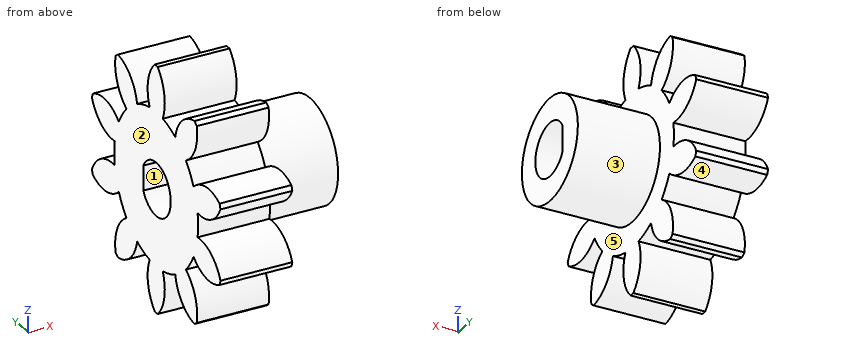
```python
from build123d import *

# Parameters (mm, degrees)
BASPROSKE_W         = 15
BASPROSKE_H         = 12
TOOTHCUT_DEPTH      = 23.649503306
TEETHCUTS_COUNT     = 10
TEETHCUTS_ANGLE     = 324
BORSKE_R            = 0.45
BORE_DEPTH          = 50.0000508
SKETCH1_R           = 0.45
CUT_EXTRUDE1_DEPTH  = 15
CUT_EXTRUDE2_DEPTH  = 8
SKETCH6_R           = 5
BOSS_EXTRUDE1_DEPTH = 8


with BuildPart() as part:
    # BasProSke → Base-Revolve (revolve)
    with BuildSketch(Plane(origin=(0, 0, 0), x_dir=(1, 0, 0), z_dir=(0, 1, 0)), mode=Mode.PRIVATE) as base_revolve_sk:
        with Locations((7.5, 6)):
            Rectangle(BASPROSKE_W, BASPROSKE_H)
    revolve(base_revolve_sk.sketch.rotate(Axis((-10, 0, 0), (1, 0, 0)), 180), axis=Axis((-10, 0, 0), (1, 0, 0)))

    # TooCutSke → ToothCut (cut, through all)
    with BuildSketch(Plane(origin=(0, 0, 0), x_dir=(0, 0, -1), z_dir=(1, 0, 0))):
        with BuildLine():
            ThreePointArc((1.173662691, 7.406586048), (0, 7.499), (-1.173662691, 7.406586048))
            ThreePointArc((-1.173662691, 7.406586048), (-1.668191438, 9.834565786), (-3.497907776, 11.50542856))
            ThreePointArc((-3.497907776, 11.50542856), (0, 12.0254), (3.497907776, 11.50542856))
            ThreePointArc((3.497907776, 11.50542856), (1.668191438, 9.834565786), (1.173662691, 7.406586048))
        make_face()
    toothcut = extrude(amount=TOOTHCUT_DEPTH, mode=Mode.SUBTRACT)

    # TeethCuts: ToothCut ×10 about axis
    teethcuts_axis = Axis((-10, 0, 0), (1, 0, 0))
    for i in range(1, TEETHCUTS_COUNT):
        add(toothcut.rotate(teethcuts_axis, i * TEETHCUTS_ANGLE / (TEETHCUTS_COUNT - 1)), mode=Mode.SUBTRACT)

    # BorSke → Bore (cut, symmetric)
    with BuildSketch(Plane(origin=(0, 0, 0), x_dir=(0, 0, -1), z_dir=(1, 0, 0))):
        with Locations(Location((0, 0, 0), (0, 0, 180))):
            Circle(BORSKE_R)
    extrude(amount=BORE_DEPTH, both=True, mode=Mode.SUBTRACT)

    # Sketch1 → Cut-Extrude1 (cut)
    with BuildSketch(Plane.ZY):
        with BuildLine():
            Line((1.212435565, 2.3), (-1.212435565, 2.3))
            ThreePointArc((-1.212435565, 2.3), (-1.343068786, -2.226244873), (2.6, 0))
            ThreePointArc((2.6, 0), (2.226244873, 1.343068786), (1.212435565, 2.3))
        make_face()
        Circle(SKETCH1_R, mode=Mode.SUBTRACT)
    extrude(amount=-CUT_EXTRUDE1_DEPTH, mode=Mode.SUBTRACT)

    # Sketch5 → Cut-Extrude2 (cut)
    with BuildSketch(Plane.ZY):
        with BuildLine():
            ThreePointArc((-7.406763642, 1.172541409), (-9.849931218, 1.456299749), (-11.997250213, 0.256880001))
            ThreePointArc((-11.997250213, 0.256880001), (-12, 0), (-11.997250213, -0.256880001))
            ThreePointArc((-11.997250213, -0.256880001), (-9.849931218, -1.456299749), (-7.406763642, -1.172541409))
            ThreePointArc((-7.406763642, -1.172541409), (-7.131972816, -2.317318441), (-6.681400207, -3.404980509))
            ThreePointArc((-6.681400207, -3.404980509), (-8.824753264, -4.61147306), (-9.856969584, -6.843986457))
            ThreePointArc((-9.856969584, -6.843986457), (-9.708203932, -7.053423028), (-9.554989032, -7.259627029))
            ThreePointArc((-9.554989032, -7.259627029), (-7.112770233, -6.967815552), (-5.302995112, -5.302192362))
            ThreePointArc((-5.302995112, -5.302192362), (-4.407801607, -6.066818441), (-3.403968986, -6.681915604))
            ThreePointArc((-3.403968986, -6.681915604), (-4.428819506, -8.917819898), (-3.9516616, -11.330682707))
            ThreePointArc((-3.9516616, -11.330682707), (-3.708203932, -11.412678196), (-3.463046803, -11.489443278))
            ThreePointArc((-3.463046803, -11.489443278), (-1.658772773, -9.817862641), (-1.173662691, -7.406586048))
            ThreePointArc((-1.173662691, -7.406586048), (0, -7.499), (1.173662691, -7.406586048))
            ThreePointArc((1.173662691, -7.406586048), (1.658772773, -9.817862641), (3.463046803, -11.489443278))
            ThreePointArc((3.463046803, -11.489443278), (3.708203932, -11.412678196), (3.9516616, -11.330682707))
            ThreePointArc((3.9516616, -11.330682707), (4.428819506, -8.917819898), (3.403968986, -6.681915604))
            ThreePointArc((3.403968986, -6.681915604), (4.407801607, -6.066818441), (5.302995112, -5.302192362))
            ThreePointArc((5.302995112, -5.302192362), (7.112770233, -6.967815552), (9.554989032, -7.259627029))
            ThreePointArc((9.554989032, -7.259627029), (9.708203932, -7.053423028), (9.856969584, -6.843986457))
            ThreePointArc((9.856969584, -6.843986457), (8.824753264, -4.61147306), (6.681400207, -3.404980509))
            ThreePointArc((6.681400207, -3.404980509), (7.131972816, -2.317318441), (7.406763642, -1.172541409))
            ThreePointArc((7.406763642, -1.172541409), (9.849931218, -1.456299749), (11.997250213, -0.256880001))
            ThreePointArc((11.997250213, -0.256880001), (12, 0), (11.997250213, 0.256880001))
            ThreePointArc((11.997250213, 0.256880001), (9.849931218, 1.456299749), (7.406763642, 1.172541409))
            ThreePointArc((7.406763642, 1.172541409), (7.131972816, 2.317318441), (6.681400207, 3.404980509))
            ThreePointArc((6.681400207, 3.404980509), (8.824753264, 4.61147306), (9.856969584, 6.843986457))
            ThreePointArc((9.856969584, 6.843986457), (9.708203932, 7.053423028), (9.554989032, 7.259627029))
            ThreePointArc((9.554989032, 7.259627029), (7.112770233, 6.967815552), (5.302995112, 5.302192362))
            ThreePointArc((5.302995112, 5.302192362), (4.407801607, 6.066818441), (3.403968986, 6.681915604))
            ThreePointArc((3.403968986, 6.681915604), (4.428819506, 8.917819898), (3.9516616, 11.330682707))
            ThreePointArc((3.9516616, 11.330682707), (3.708203932, 11.412678196), (3.463046803, 11.489443278))
            ThreePointArc((3.463046803, 11.489443278), (1.658772773, 9.817862641), (1.173662691, 7.406586048))
            ThreePointArc((1.173662691, 7.406586048), (0, 7.499), (-1.173662691, 7.406586048))
            ThreePointArc((-1.173662691, 7.406586048), (-1.658772773, 9.817862641), (-3.463046803, 11.489443278))
            ThreePointArc((-3.463046803, 11.489443278), (-3.708203932, 11.412678196), (-3.9516616, 11.330682707))
            ThreePointArc((-3.9516616, 11.330682707), (-4.428819506, 8.917819898), (-3.403968986, 6.681915604))
            ThreePointArc((-3.403968986, 6.681915604), (-4.407801607, 6.066818441), (-5.302995112, 5.302192362))
            ThreePointArc((-5.302995112, 5.302192362), (-7.112770233, 6.967815552), (-9.554989032, 7.259627029))
            ThreePointArc((-9.554989032, 7.259627029), (-9.708203932, 7.053423028), (-9.856969584, 6.843986457))
            ThreePointArc((-9.856969584, 6.843986457), (-8.824753264, 4.61147306), (-6.681400207, 3.404980509))
            ThreePointArc((-6.681400207, 3.404980509), (-7.131972816, 2.317318441), (-7.406763642, 1.172541409))
        make_face()
    extrude(amount=-CUT_EXTRUDE2_DEPTH, mode=Mode.SUBTRACT)

    # Sketch6 → Boss-Extrude1 (add)
    with BuildSketch(Plane(origin=(15, 0, 0), x_dir=(0, 0, -1), z_dir=(1, 0, 0))):
        with Locations(Location((0, 0, 0), (0, 0, 180))):
            Circle(SKETCH6_R)
        with BuildLine():
            Line((1.212435565, 2.3), (-1.212435565, 2.3))
            ThreePointArc((-1.212435565, 2.3), (0, -2.6), (1.212435565, 2.3))
        make_face(mode=Mode.SUBTRACT)
    extrude(amount=BOSS_EXTRUDE1_DEPTH)


solid = part.part
```
Here's how the part is built. I have some questions about the finished solid (model axes, mm). Face numbers are marked on the shaded views. A direction names the side the tool comes from. Give positions to 0.01 mm unless a question says otherwise; leave off trailing zeros. Loops run counter-clockwise (first coordinate to the right, second up) from the corner with the lowest first, then second, coordinate; pieces in that order, holes last. Notation, with made-up numbers: M 80.5,43.25 L 109.5,43.25 A23 ccw 109.5,52.25 Z; hole C -3,84.25 d11. An arc over 180 degrees is marked long. Use one line per item in the form item = value. Start each with the question number.
Q1. Thinking about a two-plate mould opening in Y: for the marked faces 3, 4 and 5, which applies, +Y half, -Y half, draft (parallel to the pull), parting line (faces both ways), or undercut?
Q2. I need wall thicknesses on line 1 along Y through (x, z) = (11.75, 0); line 2 along Y through (x, z) = (18.25, 0); line 3 along Y through (x, z) = (14.5, 8.25). Which ranges of each line are inside material? Lowest first, please.
Q3. Which directions (+Z, -Z, +X, -X, +Y, -Y) give clear straight access to the entire face, cutting with the end or side of a thin tool? Please do the marked faces 1 and 2.
Q4. If we section it at B-B (x = 18.75): Write out the boundary of the cut face in (y, z), then the cut area to 3 significant figures.
Q5. Will these pins go through, and if not, where does the flat tip stop? pin 1 Ø2 at (y, z) = (-7, 2.5) entering from +X; pin 2 Ø4.5 at (y, z) = (0, 0) entering from -X; pin 3 Ø1.2 at (x, z) = (12.5, 0) entering from -Y; pin 4 Ø6 at (x, y) = (20.5, 2.5) entering from +Z.
Q6. If we section it at A-A (z = 0): Write out the boundary of the cut face in (x, y).
Q7. If we section it at C-C (z = -9.25): Write out the boundary of the cut face in (x, y).
Q8. If we section it at D-D (y = -4): Write out the boundary of the cut face in (x, z), then the cut area to 3 significant figures.
Taken from the geometry:
q1.face_3 = parting line
q1.face_4 = undercut
q1.face_5 = draft
q2.line_1 = -7.5 to -2.6, 2.3 to 7.5
q2.line_2 = -5 to -2.6, 2.3 to 5
q2.line_3 = -7.3 to -4.1, -1.45 to 1.45, 4.1 to 7.3
q3.face_1 = +X, -X
q3.face_2 = +Z, -Z, -X, +Y, -Y
q4.outline = C 0,0 d10; hole M 2.3,-1.21 L 2.3,1.21 A2.6 ccw long Z
q4.area = 57.8 mm^2
q5.pin_1 = 15
q5.pin_2 = through
q5.pin_3 = -7.5
q5.pin_4 = 5
q6.outline = M 8,-7.5 L 15,-7.5 L 15,-5 L 23,-5 L 23,-2.6 L 8,-2.6 Z; M 8,2.3 L 23,2.3 L 23,5 L 15,5 L 15,7.5 L 8,7.5 Z
q7.outline = M 8,-7.31 L 15,-7.31 L 15,-5.16 L 8,-5.16 Z; M 8,-1.53 L 15,-1.53 L 15,1.53 L 8,1.53 Z; M 8,5.16 L 15,5.16 L 15,7.31 L 8,7.31 Z
q8.outline = M 8,-8.11 L 15,-8.11 L 15,-3 L 23,-3 L 23,3 L 15,3 L 15,8.11 L 8,8.11 Z
q8.area = 162 mm^2
